Build history of the part. All positions in model axes, mm. A direction names the side the tool comes from. Round coordinates to 2 decimals unless told otherwise and drop trailing zeros. Write each loop counter-clockwise with the first axis right and the second up, starting at its lowest first coordinate (ties: lowest second). Pieces come first, ordered by that corner, then holes.
from build123d import *

# Parameters (mm, degrees)
F0_W     = 72
F0_H     = 55
F0_R     = 2.5
F0_W_2   = 10.5
F0_H_2   = 42
F0_H_3   = 31
F1_DEPTH = 2
F2_DEPTH = 17
F3_DEPTH = 10
F4_R     = 2.5


with BuildPart() as f1:
    # F0 (on Top) → F1 (new body)
    with BuildSketch(Plane.XY):
        with Locations((36, 27.5)):
            Rectangle(F0_W, F0_H)
        with Locations((21.618534, 19.316525)):
            Circle(F0_R, mode=Mode.SUBTRACT)
        with Locations((21.576459, 26.316399)):
            Circle(F0_R, mode=Mode.SUBTRACT)
        with Locations((47.944249, 18.500125)):
            Circle(F0_R, mode=Mode.SUBTRACT)
        with Locations((47.903061, 25.500003)):
            Circle(F0_R, mode=Mode.SUBTRACT)
        with Locations((6.45, 27.5)):
            Rectangle(F0_W_2, F0_H_2, mode=Mode.SUBTRACT)
        with Locations((21.534385, 33.316272)):
            Circle(F0_R, mode=Mode.SUBTRACT)
        with Locations((21.49231, 40.316146)):
            Circle(F0_R, mode=Mode.SUBTRACT)
        with Locations((47.861874, 32.499882)):
            Circle(F0_R, mode=Mode.SUBTRACT)
        with Locations((47.820686, 39.499761)):
            Circle(F0_R, mode=Mode.SUBTRACT)
        with Locations((65.55, 27.5)):
            Rectangle(F0_W_2, F0_H_3, mode=Mode.SUBTRACT)
    extrude(amount=F1_DEPTH)

    # F0 (on Top) → F2 (join)
    with BuildSketch(Plane.XY):
        with Locations((65.55, 27.5)):
            Rectangle(F0_W_2, F0_H_3)
        with Locations((6.45, 27.5)):
            Rectangle(F0_W_2, F0_H_2)
    extrude(amount=F2_DEPTH)

    # F0 (on Top) → F3 (join)
    with BuildSketch(Plane.XY):
        with Locations((21.49231, 40.316146)):
            Circle(F0_R)
        with Locations((21.534385, 33.316272)):
            Circle(F0_R)
        with Locations((21.576459, 26.316399)):
            Circle(F0_R)
        with Locations((21.618534, 19.316525)):
            Circle(F0_R)
        with Locations((47.820686, 39.499761)):
            Circle(F0_R)
        with Locations((47.861874, 32.499882)):
            Circle(F0_R)
        with Locations((47.903061, 25.500003)):
            Circle(F0_R)
        with Locations((47.944249, 18.500125)):
            Circle(F0_R)
    extrude(amount=F3_DEPTH)

    # F4
    f4_edges = [f1.edges().sort_by_distance(p)[0] for p in [
        (18.99231, 40.316146, 10),
        (19.034385, 33.316272, 10),
        (19.076459, 26.316399, 10),
        (19.118534, 19.316525, 10),
        (45.320686, 39.499761, 10),
        (45.361874, 32.499882, 10),
        (45.403061, 25.500003, 10),
        (45.444249, 18.500125, 10),
    ]]
    fillet(f4_edges, radius=F4_R)


solid = f1.part
1) Which spindle directions (+Z, -Z, +X, -X, +Y, -Y) get a long thin tool onto all of the face, cutting with end or side? Do faces 1 (the flat face through (60.3, 27, 9)), 2 (the flat face through (1.2, 27, 9)), 3 (the flat face through (70.8, 27, 9)). Say none if no direction does.
Results:
face 1: +Z, +Y, -Y
face 2: +Z, -X, +Y, -Y
face 3: +Z, +X, +Y, -Y
2) Pin check, flat tips, straight feed: pin 1 Ø7.5 at (y, z) = (31, 7.5) entering from +X; pin 2 Ø4 at (x, z) = (28, 5.5) entering from +Y; pin 3 Ø3 at (x, z) = (8.5, 11.5) entering from +Y; pin 4 Ø8.5 at (x, z) = (64, 13) entering from +Y. Stop position of each tip, or through.
Results:
pin 1: stops at x = 70.8
pin 2: passes through
pin 3: stops at y = 48.5
pin 4: stops at y = 43
3) Slice it at C-C (y = 10). Write the cut outline in (x, z), plus the area to 4 significant figures.
Results:
outline: (0, 0) - (72, 0) - (72, 2) - (11.7, 2) - (11.7, 17) - (1.2, 17) - (1.2, 2) - (0, 2) - close
area: 301.5 mm2
4) Slice it at D-D (z = 6.5). Count the separate pieces of the cut face and the enclosed holes in it, plus the area to 3 significant figures.
Results:
separate pieces: 10
enclosed holes: 0
area: 924 mm2
5) Slice it at A-A (z = 14). Write the cut outline in (x, y), plus the area to 4 significant figures.
Results:
outline: (1.2, 6.5) - (11.7, 6.5) - (11.7, 48.5) - (1.2, 48.5) - close; (60.3, 12) - (70.8, 12) - (70.8, 43) - (60.3, 43) - close
area: 766.5 mm2
6) Wall check: L1, parallel to X at y = 16, z = 15; L2, parallel to Z at x = 35, y = 22; L3, parallel to X at y = 31.5, z = 9.5. Give the ranges that are in metal, low to high.
Results:
L1: x = 1.2 to 11.7, 60.3 to 70.8
L2: z = 0 to 2
L3: x = 1.2 to 11.7, 46.74 to 48.98, 60.3 to 70.8
7) Slice it at B-B (x = 65). Write the cut outline in (y, z).
Results:
outline: (0, 0) - (55, 0) - (55, 2) - (43, 2) - (43, 17) - (12, 17) - (12, 2) - (0, 2) - close
